Read the model definition and answer for the solid it produces. Units are mm, in the model's axes. Coordinates: 2 decimals unless noted, no trailing zeros. Write each loop counter-clockwise with the first axis right and the second up, starting at its lowest first coordinate (ties: lowest second). Pieces come first, ordered by that corner, then holes. Notation, with made-up numbers: M -7,68 L 36,68 A14 ccw 36,83 Z; hole C -30,50.25 d5. An arc over 180 degrees is marked long. Use a Markdown table: item, result. Add a question column.
from build123d import *

# Parameters (mm, degrees)
SKETCH2_W          = 76.2
SKETCH2_H          = 76.2
CUT_EXTRUDE1_DEPTH = 13.97


with BuildPart() as part:
    # Sketch1 → Revolve1 (revolve)
    with BuildSketch(Plane(origin=(0, 0, 0), x_dir=(0, 0, -1), z_dir=(1, 0, 0))):
        Polygon((0, 0), (0, 19.05), (1.020886423, 22.86), (12.949113577, 22.86), (13.97, 19.05), (13.97, 0), align=None)
    revolve(axis=Axis((0, 0, -13.97), (0, 0, 1)))

    # Sketch2 → Cut-Extrude1 (cut)
    with BuildSketch(Plane.XY):
        Rectangle(SKETCH2_W, SKETCH2_H)
        Polygon((-19.05, 10.998522628), (-19.05, -10.998522628), (0, -21.997045256), (19.05, -10.998522628), (19.05, 10.998522628), (0, 21.997045256), align=None, mode=Mode.SUBTRACT)
    extrude(amount=-CUT_EXTRUDE1_DEPTH, mode=Mode.SUBTRACT)

    # Sketch3 → Cut-Revolve1 (revolve, cut)
    with BuildSketch(Plane(origin=(0, 0, 0), x_dir=(0, 0, -1), z_dir=(1, 0, 0))):
        Polygon((0, 0), (0, 12.7), (0.9779, 11.7221), (12.9921, 11.7221), (13.97, 12.7), (13.97, 0), align=None)
    revolve(axis=Axis((0, 0, -13.97), (0, 0, 1)), mode=Mode.SUBTRACT)


solid = part.part
Item 1: Find section A-A on z = -7.5. Give the vertices of the cut face in (x, y), then the cut area to 3 significant figures.
Item 2: Determine the mould class of faces 1 (the flat face through (19.05, 0, -7)), 2 (the conical face through (-17.08, 9.92, -13.78)), 3 (the conical face through (17.09, -9.92, -0.19)), 4 (the cylindrical face through (-11.62, -1.53, -7.07)) for opening direction Y: pulls with the +Y half, pulls with the -Y half, needs draft (parallel to the pull), parting line crosses it, or undercut.
Item 3: Each of these flat-tipped pins is pushed along its axis until it touches: pin 1 (4 mm diameter, centred on x = -2.5, z = -11.5, fed in from -Y); pin 2 (2 mm diameter, centred on x = 7, z = -8.5, fed in from +Y); pin 3 (1 mm diameter, centred on x = 10.5, z = -11, fed in from +Y). Where does it stop, or does it pass through?
Item 4: Consider probe 1 along Y at (x, z) = (0, -3.5); probe 2 along Y at (x, z) = (7.5, -9.25); probe 3 along X at (y, z) = (-0.5, -7.5). Determine where each line is inside the solid, lowest interval first.
Geometry says:
| question | item | result |
|---|---|---|
| 1 | outline | M -19.05,-11 L 0,-22 L 19.05,-11 L 19.05,11 L 0,22 L -19.05,11 Z; hole C 0,0 d23.44 |
| 1 | area | 825 mm2 |
| 2 | face 1 | needs draft |
| 2 | face 2 | pulls with the +Y half |
| 2 | face 3 | pulls with the -Y half |
| 2 | face 4 | undercut |
| 3 | pin 1 | stops at y = -21.71 |
| 3 | pin 2 | stops at y = 18.53 |
| 3 | pin 3 | stops at y = 16.22 |
| 4 | probe 1 | y = -22 to -11.72, 11.72 to 22 |
| 4 | probe 2 | y = -17.67 to -9.01, 9.01 to 17.67 |
| 4 | probe 3 | x = -19.05 to -11.71, 11.71 to 19.05 |
